```python
from build123d import *

# Parameters (mm, degrees)
SKETCH1_W           = 32.526911934
SKETCH1_H           = 32.526911934
BOSS_EXTRUDE1_DEPTH = 4
FILLET1_R           = 4
CHAMFER1_SIZE       = 2
SKETCH2_R           = 1
CUT_EXTRUDE1_DEPTH  = 24.34523506


with BuildPart() as part:
    # Sketch1 → Boss-Extrude1 (new body)
    with BuildSketch(Plane.XY):
        Rectangle(SKETCH1_W, SKETCH1_H)
    extrude(amount=BOSS_EXTRUDE1_DEPTH)

    # Fillet1
    fillet1_edges = [part.edges().sort_by_distance(p)[0] for p in [
        (-16.263455967, 16.263455967, 2),
        (16.263455967, 16.263455967, 2),
        (16.263455967, -16.263455967, 2),
        (-16.263455967, -16.263455967, 2),
    ]]
    fillet(fillet1_edges, radius=FILLET1_R)

    # Chamfer1
    chamfer1_edges = [part.edges().sort_by_distance(p)[0] for p in [
        (0, -16.263455967, 4),
        (-16.263455967, 0, 4),
        (16.263455967, 0, 4),
        (0, 16.263455967, 4),
        (-15.091883092, 15.091883092, 4),
        (15.091883092, 15.091883092, 4),
        (15.091883092, -15.091883092, 4),
        (-15.091883092, -15.091883092, 4),
    ]]
    chamfer(chamfer1_edges, length=CHAMFER1_SIZE)

    # Sketch2 → Cut-Extrude1 (cut, through all)
    with BuildSketch(Plane.XY.offset(4)):
        Circle(SKETCH2_R)
    extrude(amount=-CUT_EXTRUDE1_DEPTH, mode=Mode.SUBTRACT)


solid = part.part
```
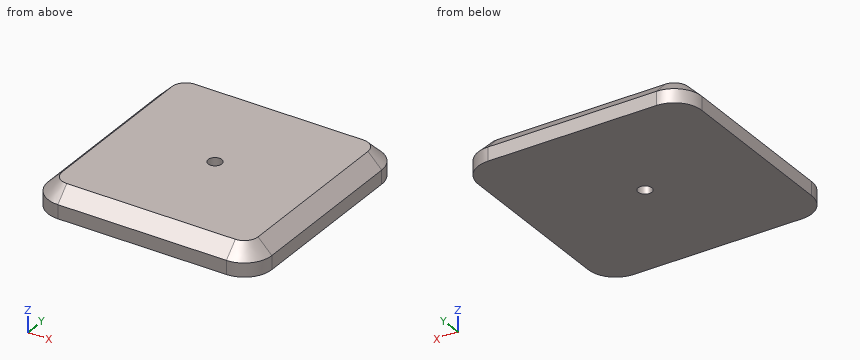
Verification items for the finished model (mm, model axes). Round coordinates to 2 decimals unless told otherwise and drop trailing zeros. Loops run counter-clockwise (first coordinate to the right, second up) from the corner with the lowest first, then second, coordinate; pieces in that order, holes last. Notation, with made-up numbers: (55.25, 23.5) -> (100.25, 23.5) arc R22 ccw to (100.25, 39.5) -> close; hole circle Ø2 at (-0.75, -13.75). An arc over 180 degrees is marked (long way). Answer as a JSON object with one key per item and string values.
Q1. Section check A-A (z = 0.9). Record the boundary of the cut face in (x, y).
Data:
{"outline": "(-16.26, -12.26) arc R4 ccw to (-12.26, -16.26) -> (12.26, -16.26) arc R4 ccw to (16.26, -12.26) -> (16.26, 12.26) arc R4 ccw to (12.26, 16.26) -> (-12.26, 16.26) arc R4 ccw to (-16.26, 12.26) -> close; hole circle Ø2 at (0, 0)"}
Q2. Scan lines: line 1 (Y direction, x = 0, z = 1.25); line 2 (Y direction, x = 0, z = 2.5); line 3 (X direction, y = 1.5, z = 3.7). Record each from-to range of solid material in increasing order. Write a range as from..to.
Data:
{"line 1": "y = -16.26..-1, 1..16.26", "line 2": "y = -15.76..-1, 1..15.76", "line 3": "x = -14.56..14.56"}
Q3. Section check B-B (y = 0). Record the boundary of the cut face in (x, z), then the cut area to 3 significant figures.
Data:
{"outline": "(-16.26, 0) -> (-1, 0) -> (-1, 4) -> (-14.26, 4) -> (-16.26, 2) -> close; (1, 0) -> (16.26, 0) -> (16.26, 2) -> (14.26, 4) -> (1, 4) -> close", "area": "118 mm2"}
